Study the drawing (mm; zero at the part's minimum x, y, z) and answer. Coordinates: 2 decimals unless noted, no trailing zeros. Order: outer loops, then holes, each group sorted by start corner. A loop starts at its lowest first (then second) coordinate and runs counter-clockwise, first axis right, second up.
1. The part is cut by section B-B, the plane x = 24.13. Give the vertices of the cut face in (y, z).
2. The part is cut by section C-C, the plane z = 3.75. Count the separate pieces of the cut face and the enclosed holes in it, then the cut area to 3 significant figures.
3. Find the intervals of material crossed by probe 1 along Y at (x, z) = (88.9, 4) (1 decimal); probe 2 along Y at (x, z) = (24.13, 4); probe 3 along X at (y, z) = (9.5, 5.25) (1 decimal), in increasing order.
4. Flat-ended cylindrical pins translate along their axes: pin 1 Ø6 at (x, y) = (24.13, 8.001) entering from +Z; pin 2 Ø4 at (x, y) = (161.65, 8) entering from +Z; pin 3 Ø1.5 at (x, z) = (45, 5) entering from +Y. Find the tip coordinate at first contact, or state that the pin passes through.
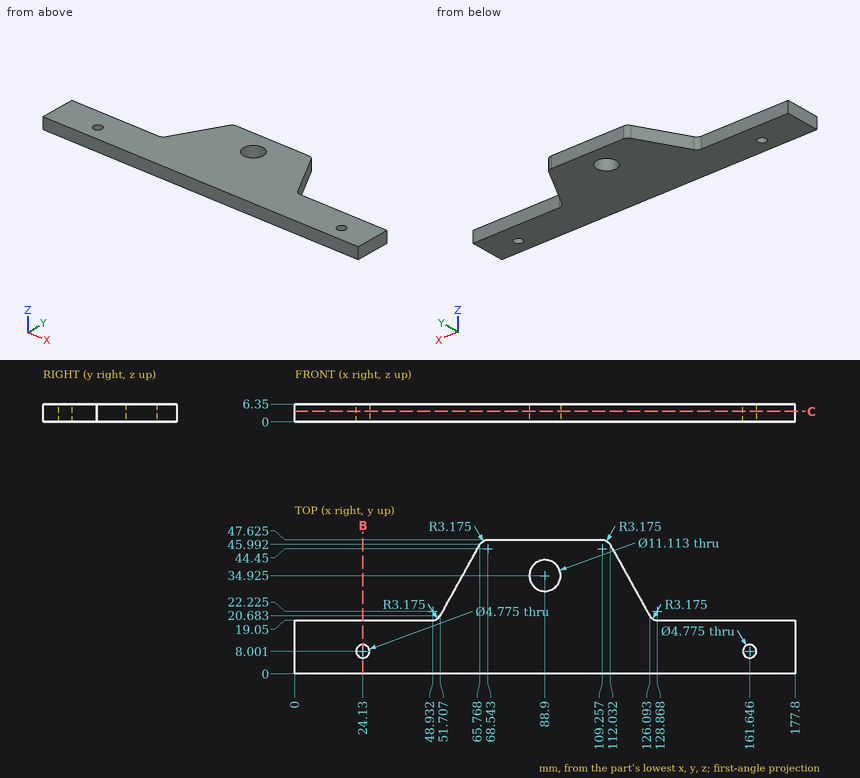
Geometry says:
1. outline: (0, 0) - (5.61, 0) - (5.61, 6.35) - (0, 6.35) - close; (10.39, 0) - (19.05, 0) - (19.05, 6.35) - (10.39, 6.35) - close
2. separate pieces: 1
2. enclosed holes: 3
2. area: 4,980 mm2
3. probe 1: y = 0 to 29.4, 40.5 to 47.6
3. probe 2: y = 0 to 5.61, 10.39 to 19.05
3. probe 3: x = 0 to 22.3, 26 to 159.8, 163.5 to 177.8
4. pin 1: stops at z = 6.35
4. pin 2: passes through
4. pin 3: stops at y = 19.05
